from build123d import *

# Parameters (mm, degrees)
F0_W     = 25
F0_H     = 25
F2_DEPTH = 30
F3_W     = 17.673826
F3_H     = 9.68429
F4_DEPTH = 9
F5_R     = 1.434881
F6_DEPTH = 10


with BuildPart() as f2:
    # F0 (on Top) → F2 (new body)
    with BuildSketch(Plane.XY):
        Rectangle(F0_W, F0_H)
    extrude(amount=F2_DEPTH)

    # F3 (on face) → F4 (cut)
    with BuildSketch(Plane.XZ.offset(12.5)):
        with Locations((-0.060834, 19.375956)):
            Rectangle(F3_W, F3_H)
    extrude(amount=-F4_DEPTH, mode=Mode.SUBTRACT)

    # F5 (on offset) → F6 (join)
    with BuildSketch(Plane.XY.offset(30)):
        with Locations((-3.82385, -3.980379)):
            Circle(F5_R)
        with Locations((3.82385, -3.980379)):
            Circle(F5_R)
    extrude(amount=-F6_DEPTH)


solid = f2.part
Design review of the part built by this model. Coordinates are the model's own, in mm. A direction names the side the tool comes from. Coordinates: 2 decimals unless noted, no trailing zeros. Write each loop counter-clockwise with the first axis right and the second up, starting at its lowest first coordinate (ties: lowest second). Pieces come first, ordered by that corner, then holes. Notation, with made-up numbers: (37.5, 63.25) - (75.5, 63.25) arc R9 ccw to (75.5, 67.25) - close; hole circle Ø7 at (57, 41). An arc over 180 degrees is marked (long way). Use one line per item in the form item = value.
Q1. Consider section A-A (y = -8.5). Write out the cut boundary in (x, z).
Taken from the geometry:
outline = (-12.5, 0) - (12.5, 0) - (12.5, 30) - (-12.5, 30) - close; hole (-8.9, 14.53) - (8.78, 14.53) - (8.78, 24.22) - (-8.9, 24.22) - close
Q2. Machinability: for faces 1 (the flat face through (-12.5, 0, 15)), 2 (the cylindrical face through (3.785, -5.415, 22.139)), 3 (the flat face through (-8.898, -8, 19)), which of the approach directions +Z, -Z, +X, -X, +Y, -Y give a long, thin tool a straight path to every point of the face, cutting with its end or side? Answer none if there is none.
Taken from the geometry:
face_1 = +Z, -Z, -X, +Y, -Y
face_2 = none
face_3 = -Y
Q3. The part is to be moulded in two halves that separate along Z. For faces 4 (the cylindrical face through (-3.862, -5.415, 22.139)), 5 (the flat face through (0, 0, 30)), 6 (the flat face through (0, 12.5, 15)), say which applies: +Z half, -Z half, draft (parallel to the pull), parting line (faces both ways), or undercut.
Taken from the geometry:
face_4 = undercut
face_5 = +Z half
face_6 = draft
Q4. Consider section B-B (x = 8). Write out the cut boundary in (y, z), plus the area to 3 significant figures.
Taken from the geometry:
outline = (-12.5, 0) - (12.5, 0) - (12.5, 30) - (-12.5, 30) - (-12.5, 24.22) - (-3.5, 24.22) - (-3.5, 14.53) - (-12.5, 14.53) - close
area = 663 mm^2
Q5. For probe 1 along Z at (x, y) = (6.5, -4.5); probe 2 along Z at (x, y) = (4.25, -4.5); probe 3 along Y at (x, z) = (2, 17.5), list the stretches that pass through material, from the lowest coordinate up.
Taken from the geometry:
probe_1 = 0 to 14.53, 24.22 to 30
probe_2 = 0 to 14.53, 20 to 30
probe_3 = -3.5 to 12.5
Q6. Insertion check: pin 1 Ø1.5 at (x, y) = (-4, -5) entering from -Z; pin 2 Ø5 at (x, z) = (4, 19.5) entering from -Y; pin 3 Ø3 at (x, z) = (7, 16.5) entering from -Y. Each pin has a flat end and moves straight along its axis. Give the tip position at first contact, or say it passes through.
Taken from the geometry:
pin_1 = 0
pin_2 = -5.42
pin_3 = -3.5
Q7. Consider section C-C (z = 15). Write out the cut boundary in (x, y), plus the area to 3 significant figures.
Taken from the geometry:
outline = (-12.5, -12.5) - (-8.9, -12.5) - (-8.9, -3.5) - (8.78, -3.5) - (8.78, -12.5) - (12.5, -12.5) - (12.5, 12.5) - (-12.5, 12.5) - close
area = 466 mm^2
Q8. Consider section D-D (y = -4). Write out the cut boundary in (x, z).
Taken from the geometry:
outline = (-12.5, 0) - (12.5, 0) - (12.5, 30) - (-12.5, 30) - close; hole (-8.9, 14.53) - (8.78, 14.53) - (8.78, 24.22) - (5.26, 24.22) - (5.26, 20) - (2.39, 20) - (2.39, 24.22) - (-2.39, 24.22) - (-2.39, 20) - (-5.26, 20) - (-5.26, 24.22) - (-8.9, 24.22) - close
